from build123d import *

# Parameters (mm, degrees)
SKETCH1_R           = 1.4605
SKETCH1_R_2         = 0.4318
SKETCH1_W           = 85.0392
SKETCH1_H           = 55.626
BOSS_EXTRUDE1_DEPTH = 1.6256
SKETCH1_2_W         = 85.0392
SKETCH1_2_H         = 55.626
BOSS_EXTRUDE2_DEPTH = 5.334
SKETCH2_W           = 57.3786
SKETCH2_H           = 56.134
BOSS_EXTRUDE3_DEPTH = 2.54


with BuildPart() as part:
    # Sketch1 → Boss-Extrude1 (new body)
    with BuildSketch(Plane(origin=(0, 0, 0), x_dir=(1, 0, 0), z_dir=(0, 1, 0))):
        with BuildLine():
            Line((43.2943, 28.067), (-43.2943, 28.067))
            Line((-43.2943, 28.067), (-43.2943, 30.48))
            ThreePointArc((-43.2943, 30.48), (-45.8343, 33.02), (-48.3743, 30.48))
            Line((-48.3743, 30.48), (-48.3743, -30.48))
            ThreePointArc((-48.3743, -30.48), (-45.8343, -33.02), (-43.2943, -30.48))
            Line((-43.2943, -30.48), (-43.2943, -28.067))
            Line((-43.2943, -28.067), (43.2943, -28.067))
            Line((43.2943, -28.067), (43.2943, -30.48))
            ThreePointArc((43.2943, -30.48), (45.8343, -33.02), (48.3743, -30.48))
            Line((48.3743, -30.48), (48.3743, 30.48))
            ThreePointArc((48.3743, 30.48), (45.8343, 33.02), (43.2943, 30.48))
            Line((43.2943, 30.48), (43.2943, 28.067))
        make_face()
        with Locations((-45.8343, 30.48)):
            Circle(SKETCH1_R, mode=Mode.SUBTRACT)
        with Locations((-45.8343, -30.48)):
            Circle(SKETCH1_R, mode=Mode.SUBTRACT)
        with Locations((45.8343, -30.48)):
            Circle(SKETCH1_R, mode=Mode.SUBTRACT)
        with Locations((45.8343, 30.48)):
            Circle(SKETCH1_R, mode=Mode.SUBTRACT)
        with Locations((-45.8343, 24.13)):
            Circle(SKETCH1_R_2, mode=Mode.SUBTRACT)
        with Locations((-45.8343, 21.59)):
            Circle(SKETCH1_R_2, mode=Mode.SUBTRACT)
        with Locations((-45.8343, 19.05)):
            Circle(SKETCH1_R_2, mode=Mode.SUBTRACT)
        with Locations((-45.8343, 16.51)):
            Circle(SKETCH1_R_2, mode=Mode.SUBTRACT)
        with Locations((-45.8343, 13.97)):
            Circle(SKETCH1_R_2, mode=Mode.SUBTRACT)
        with Locations((-45.8343, 11.43)):
            Circle(SKETCH1_R_2, mode=Mode.SUBTRACT)
        with Locations((-45.8343, 8.89)):
            Circle(SKETCH1_R_2, mode=Mode.SUBTRACT)
        with Locations((-45.8343, 6.35)):
            Circle(SKETCH1_R_2, mode=Mode.SUBTRACT)
        with Locations((-45.8343, 3.81)):
            Circle(SKETCH1_R_2, mode=Mode.SUBTRACT)
        with Locations((-45.8343, 1.27)):
            Circle(SKETCH1_R_2, mode=Mode.SUBTRACT)
        with Locations((-45.8343, -1.27)):
            Circle(SKETCH1_R_2, mode=Mode.SUBTRACT)
        with Locations((-45.8343, -3.81)):
            Circle(SKETCH1_R_2, mode=Mode.SUBTRACT)
        with Locations((-45.8343, -6.35)):
            Circle(SKETCH1_R_2, mode=Mode.SUBTRACT)
        with Locations((-45.8343, -8.89)):
            Circle(SKETCH1_R_2, mode=Mode.SUBTRACT)
        with Locations((-45.8343, -11.43)):
            Circle(SKETCH1_R_2, mode=Mode.SUBTRACT)
        with Locations((-45.8343, -13.97)):
            Circle(SKETCH1_R_2, mode=Mode.SUBTRACT)
        with Locations((-45.8343, -16.51)):
            Circle(SKETCH1_R_2, mode=Mode.SUBTRACT)
        with Locations((-45.8343, -19.05)):
            Circle(SKETCH1_R_2, mode=Mode.SUBTRACT)
        with Locations((-45.8343, -21.59)):
            Circle(SKETCH1_R_2, mode=Mode.SUBTRACT)
        with Locations((-45.8343, -24.13)):
            Circle(SKETCH1_R_2, mode=Mode.SUBTRACT)
        with Locations((45.8343, -24.13)):
            Circle(SKETCH1_R_2, mode=Mode.SUBTRACT)
        with Locations((45.8343, -21.59)):
            Circle(SKETCH1_R_2, mode=Mode.SUBTRACT)
        with Locations((45.8343, -19.05)):
            Circle(SKETCH1_R_2, mode=Mode.SUBTRACT)
        with Locations((45.8343, -16.51)):
            Circle(SKETCH1_R_2, mode=Mode.SUBTRACT)
        with Locations((45.8343, -13.97)):
            Circle(SKETCH1_R_2, mode=Mode.SUBTRACT)
        with Locations((45.8343, -11.43)):
            Circle(SKETCH1_R_2, mode=Mode.SUBTRACT)
        with Locations((45.8343, -8.89)):
            Circle(SKETCH1_R_2, mode=Mode.SUBTRACT)
        with Locations((45.8343, -6.35)):
            Circle(SKETCH1_R_2, mode=Mode.SUBTRACT)
        with Locations((45.8343, -3.81)):
            Circle(SKETCH1_R_2, mode=Mode.SUBTRACT)
        with Locations((45.8343, -1.27)):
            Circle(SKETCH1_R_2, mode=Mode.SUBTRACT)
        with Locations((45.8343, 1.27)):
            Circle(SKETCH1_R_2, mode=Mode.SUBTRACT)
        with Locations((45.8343, 3.81)):
            Circle(SKETCH1_R_2, mode=Mode.SUBTRACT)
        with Locations((45.8343, 6.35)):
            Circle(SKETCH1_R_2, mode=Mode.SUBTRACT)
        with Locations((45.8343, 8.89)):
            Circle(SKETCH1_R_2, mode=Mode.SUBTRACT)
        with Locations((45.8343, 11.43)):
            Circle(SKETCH1_R_2, mode=Mode.SUBTRACT)
        with Locations((45.8343, 13.97)):
            Circle(SKETCH1_R_2, mode=Mode.SUBTRACT)
        with Locations((45.8343, 16.51)):
            Circle(SKETCH1_R_2, mode=Mode.SUBTRACT)
        with Locations((45.8343, 19.05)):
            Circle(SKETCH1_R_2, mode=Mode.SUBTRACT)
        with Locations((45.8343, 21.59)):
            Circle(SKETCH1_R_2, mode=Mode.SUBTRACT)
        with Locations((45.8343, 24.13)):
            Circle(SKETCH1_R_2, mode=Mode.SUBTRACT)
        Rectangle(SKETCH1_W, SKETCH1_H, mode=Mode.SUBTRACT)
    extrude(amount=BOSS_EXTRUDE1_DEPTH)

    # Sketch1<2> → Boss-Extrude2 (add)
    with BuildSketch(Plane(origin=(0, 0, 0), x_dir=(1, 0, 0), z_dir=(0, 1, 0))):
        Rectangle(SKETCH1_2_W, SKETCH1_2_H)
    extrude(amount=BOSS_EXTRUDE2_DEPTH)

    # Sketch2 → Boss-Extrude3 (add)
    with BuildSketch(Plane.XZ):
        with Locations((-5.715, 0)):
            Rectangle(SKETCH2_W, SKETCH2_H)
    extrude(amount=BOSS_EXTRUDE3_DEPTH)


solid = part.part
Geometry check sheet. Reference: the model listing, model coordinates, mm. A direction names the side the tool comes from. Round coordinates to 2 decimals unless told otherwise and drop trailing zeros. Write each loop counter-clockwise with the first axis right and the second up, starting at its lowest first coordinate (ties: lowest second). Pieces come first, ordered by that corner, then holes. Notation, with made-up numbers: (64, 65.5) -> (100, 65.5) arc R21 cw to (100, 78.5) -> close; hole circle Ø5 at (0, 18.25). An arc over 180 degrees is marked (long way). One line per item, written item: value. Start each with the question number.
(1) Scan lines: line 1 (X direction, y = 1.25, z = -21.59); line 2 (Z direction, x = 22, y = 4.5); line 3 (Y direction, x = 36.5, z = -8). Record each from-to range of solid material in increasing order. Write a range as [from, to].
(2) Access from +Z, -Z, +X, -X, +Y, -Y to the whole of each face (thin tool, end or side, straight path). Record for faces 4 (the flat face through (-1, 3, 27.813)), 5 (the flat face through (1, 0, -28.067)), 6 (the flat face through (-1, 3, -27.813)).
(3) Cross-section at A-A, the plane x = -19. Record the cut outline in (y, z).
(4) Cross-section at B-B, the plane z = -26. Record the cut outline in (x, y), and give its area (3 significant figures).
(5) Draft check along X on faces 1 (the cylindrical face through (-45.78, 0.8, -33.02)), 2 (the flat face through (22.974, -1, 0)), 3 (the flat face through (-43, 1.626, 0)). Enter one of: +X half, -X half, draft (parallel to the pull), parting line (faces both ways), or undercut.
(6) Go/stop test with flat-tipped pins: pin 1 Ø4 at (x, z) = (-38, -8) entering from -Y; pin 2 Ø3 at (x, y) = (-9, 3.5) entering from -Z; pin 3 Ø1.1 at (x, y) = (6, 2.5) entering from +Z. Record where each tip stops, or that it passes through.
(7) Cross-section at C-C, the plane x = -41.5. Record the cut outline in (y, z).
Answer:
1. line 1: [-48.37, -46.27], [-45.4, 45.4], [46.27, 48.37]
1. line 2: [-27.81, 27.81]
1. line 3: [0, 5.33]
2. face 4: +Z, +X, -X, +Y
2. face 5: -Z, +Y, -Y
2. face 6: -Z, +X, -X, +Y
3. outline: (-2.54, -28.07) -> (1.63, -28.07) -> (1.63, -27.81) -> (5.33, -27.81) -> (5.33, 27.81) -> (1.63, 27.81) -> (1.63, 28.07) -> (-2.54, 28.07) -> close
4. outline: (-48.37, 0) -> (-34.4, 0) -> (-34.4, -2.54) -> (22.97, -2.54) -> (22.97, 0) -> (48.37, 0) -> (48.37, 1.63) -> (42.52, 1.63) -> (42.52, 5.33) -> (-42.52, 5.33) -> (-42.52, 1.63) -> (-48.37, 1.63) -> close
4. area: 618 mm²
5. face 1: undercut
5. face 2: +X half
5. face 3: draft
6. pin 1: y = 0
6. pin 2: z = -27.81
6. pin 3: z = 27.81
7. outline: (0, -28.07) -> (1.63, -28.07) -> (1.63, -27.81) -> (5.33, -27.81) -> (5.33, 27.81) -> (1.63, 27.81) -> (1.63, 28.07) -> (0, 28.07) -> close
